Autodesk Inventor part; units mm, degrees
ref_plane "YZ Plane" through (0, 0, 0) normal (1, 0, 0) x (0, 1, 0)
ref_plane "XZ Plane" through (0, 0, 0) normal (0, 1, 0) x (-1, 0, 0)
ref_plane "XY Plane" through (0, 0, 0) normal (0, 0, 1) x (1, 0, 0)
sketch "Sketch1" plane through (0, 0, 0) normal (0, 1, 0) x (-1, 0, 0)
  circle A0 centre (0, -75) radius 227.5
  circle A1 centre (0, -75) radius 312.5
  line L0 (214.7819, -150) -> (303.3665, -150)
  line L1 (214.7819, 0) -> (303.3665, 0)
  line L2 (437.5, 0) -> (-437.5, 0)
  line L3 (259.0742, 0) -> (259.0742, -150) construction
  line L4 (0, 0) -> (0, -75)
  dimension "d0" = 455
  dimension "d1" = 625
  dimension "d4" = 150
  dimension "d5" = 75
extrude "Extrusion1" add sketch "Sketch1" along normal blind 10 contours A0 L1 A1 L0
sketch "Sketch2" plane through (0, 10, 0) normal (0, 1, 0) x (1, 0, 0)
  arc A0 (-214.7819, 150) -> (-214.7819, 0) centre (0, 75) ccw
  line L0 (-214.7819, 150) -> (-303.3665, 150)
  arc A1 (-303.3665, 150) -> (-303.3665, 0) centre (0, 75) ccw
  line L1 (-303.3665, 0) -> (-214.7819, 0)
  line L2 (-227.5, 75) -> (-312.5, 75) construction
  line L3 (-270, 75) -> (-270, 150) construction
  line L4 (-270, 75) -> (-270, 0) construction
  line L5 (-295, 25) -> (-245, 25)
  line L6 (-245, 25) -> (-245, 125)
  line L7 (-245, 125) -> (-295, 125)
  line L8 (-295, 125) -> (-295, 25)
  line L9 (-295, 75) -> (-245, 75) construction
  line L10 (-270, 25) -> (-270, 125) construction
  line L11 (-295, 25) -> (-295, 15) construction
  line L12 (-245, 25) -> (-245, 15) construction
  line L13 (-245, 25) -> (-235, 25) construction
  line L14 (-245, 15) -> (-230, 15) construction
  line L15 (-245, 125) -> (-245, 135) construction
  line L16 (-245, 135) -> (-230, 135) construction
  line L17 (-295, 125) -> (-295, 135) construction
  circle A2 centre (-295, 15) radius 5
  circle A3 centre (-230, 15) radius 5
  circle A4 centre (-230, 135) radius 5
  circle A5 centre (-295, 135) radius 5
  point P0 (0, 0)
  dimension "d8" = 50
  dimension "d9" = 100
  dimension "d10" = 10
  dimension "d11" = 10
  dimension "d12" = 90
  dimension "d13" = 15
  dimension "d14" = 10
  dimension "d15" = 15
  dimension "d16" = 90
  dimension "d17" = 10
  dimension "d18" = 10
  dimension "d19" = 10
  dimension "d20" = 10
  dimension "d21" = 10
extrude "Extrusion2" add sketch "Sketch2" along normal blind 40 contours A2 | A3 | A4 | A5
fillet "Fillet1" radius 10 2 edges at (-259.0742, 0, 0) (-259.0742, 0, -150)
properties part number "Battery Cage Spring Plate Second Iteration" material "PLA 33 Plastic"
Work out the finished part from the listing and answer in its coordinate system (mm). A direction names the side the tool comes from. Round coordinates to 2 decimals unless told otherwise and drop trailing zeros. Loops run counter-clockwise (first coordinate to the right, second up) from the corner with the lowest first, then second, coordinate; pieces in that order, holes last. Notation, with made-up numbers: M -29.5,-12 L 20.5,-12 A10 ccw 20.5,5 Z; hole C 18,56.25 d11. An arc over 180 degrees is marked long. One line per question, with ' | ' between items.
Q1. A tool of negligible diameter and unlimited length cuts with its end or side. For faces 4 (the cylindrical face through (-227.497, 4.93, -73.93)), 5 (the cylindrical face through (-225.23, 29.72, -133.5)), from which of +Z, -Z, +X, -X, +Y, -Y can it reach the whole face along a straight path? Write none if from no direction.
Conclusion:
face 4: +X, +Y, -Y | face 5: +Y
Q2. Find section B-B, the plane z = -135. Give the vertices of the cut face in (x, y).
Conclusion:
outline: M -306.69,0 L -219.45,0 L -219.45,10 L -225,10 L -225,50 L -235,50 L -235,10 L -290,10 L -290,50 L -300,50 L -300,10 L -306.69,10 Z
Q3. Find section C-C, the plane y = 4. Give the vertices of the cut face in (x, z).
Conclusion:
outline: M -303.85,-148 L -215.47,-148 A227.5 cw -215.47,-2 L -303.85,-2 A312.5 ccw Z
Q4. The mould has two halves that part along Z. Classify faces 1 (the cylindrical face through (-312.5, 4.9, -73.9)), 2 (the flat face through (-295, 50, -135)), 3 (the cylindrical face through (-225.23, 29.72, -13.5)): +Z half, -Z half, draft (parallel to the pull), parting line (faces both ways), or undercut.
Conclusion:
face 1: parting line | face 2: draft | face 3: undercut
Q5. Consider line 1 along Z through (x, y) = (-230.5, 32); line 2 along Y through (x, z) = (-240, -90); line 3 along Z through (x, y) = (-232, 32). Determine where each line is inside the solid, lowest interval first. Write a range as from..to.
Conclusion:
line 1: z = -139.97..-130.03, -19.97..-10.03 | line 2: y = 0..10 | line 3: z = -139.58..-130.42, -19.58..-10.42
Q6. Each of these flat-tipped pins is pushed along its axis until it touches: pin 1 Ø4 at (x, z) = (-224.5, -41.5) entering from +Y; pin 2 Ø3 at (y, z) = (6, -20.5) entering from -X; pin 3 Ø3 at (y, z) = (26.5, -133.5) entering from -X. Where does it stop, or does it pass through?
Conclusion:
pin 1: stops at y = 10 | pin 2: stops at x = -307.97 | pin 3: stops at x = -300
